```python
from build123d import *

# Parameters (mm, degrees)
F_35MM_DEPTH          = 35
CUT_EXTRUDE_1_REACH   = 50.244
SKETCH_2_R            = 10.5
FILLET_1_R            = 1
SKETCH_3_R            = 1.75
CUT_EXTRUDE_3_1_DEPTH = 35


with BuildPart() as part:
    # 草图1 → 高35mm (new body)
    with BuildSketch(Plane(origin=(0, 0, 0), x_dir=(1, 0, 0), z_dir=(0, 1, 0))):
        with BuildLine():
            Line((-20, 13.25250025), (-20, -7.909163894))
            ThreePointArc((-20, -7.909163894), (-19.67340752, -9.004475389), (-18.800292729, -9.742066387))
            ThreePointArc((-18.800292729, -9.742066387), (-16.040253129, -11.142625499), (-13.460543724, -12.852737719))
            ThreePointArc((-13.460543724, -12.852737719), (-12.893128183, -13.149929424), (-12.260860414, -13.25250025))
            Line((-12.260860414, -13.25250025), (12.260860414, -13.25250025))
            ThreePointArc((12.260860414, -13.25250025), (12.893128183, -13.149929424), (13.460543724, -12.852737719))
            ThreePointArc((13.460543724, -12.852737719), (16.040253129, -11.142625499), (18.800292729, -9.742066387))
            ThreePointArc((18.800292729, -9.742066387), (19.67340752, -9.004475389), (20, -7.909163894))
            Line((20, -7.909163894), (20, 13.25250025))
            Line((20, 13.25250025), (-20, 13.25250025))
        make_face()
    extrude(amount=F_35MM_DEPTH)

    # 草图2 → 切除-拉伸1 (cut, up to next)
    with BuildSketch(Plane(origin=(0, 0, -13.25250025), x_dir=(-1, 0, 0), z_dir=(0, 0, -1)), mode=Mode.PRIVATE) as cut_extrude_1_sk1:
        with Locations((0, 15)):
            Circle(SKETCH_2_R)
    cut_extrude_1_tool1 = extrude(cut_extrude_1_sk1.sketch, amount=-CUT_EXTRUDE_1_REACH, mode=Mode.PRIVATE) & part.part
    add(cut_extrude_1_tool1.solids().sort_by_distance((0, 15, -13.2525))[0], mode=Mode.SUBTRACT)

    # 圆角1
    fillet_1_edges = [part.edges().sort_by_distance(p)[0] for p in [
        (10.5, 15, -13.25250025),
        (10.5, 15, 13.25250025),
    ]]
    fillet(fillet_1_edges, radius=FILLET_1_R)

    # 草图3 → φ3.1通孔 (cut)
    with BuildSketch(Plane(origin=(0, 35, 0), x_dir=(1, 0, 0), z_dir=(0, 1, 0))):
        with Locations(Location((-15, 8.25250025, 0), (0, 0, 270))):
            Circle(SKETCH_3_R)
        with Locations(Location((-15, -6.74749975, 0), (0, 0, 270))):
            Circle(SKETCH_3_R)
        with Locations(Location((15, -6.74749975, 0), (0, 0, 90))):
            Circle(SKETCH_3_R)
        with Locations(Location((15, 8.25250025, 0), (0, 0, 90))):
            Circle(SKETCH_3_R)
    extrude(amount=-CUT_EXTRUDE_3_1_DEPTH, mode=Mode.SUBTRACT)


solid = part.part
```
Build history of the part. All positions in model axes, mm. Give positions to 0.01 mm unless a question says otherwise; leave off trailing zeros. Loops run counter-clockwise (first coordinate to the right, second up) from the corner with the lowest first, then second, coordinate; pieces in that order, holes last. Notation, with made-up numbers: (-37.5, 78.25) -> (10.5, 78.25) arc R20 ccw to (10.5, 82.25) -> close; hole circle Ø6 at (-3.5, 5). An arc over 180 degrees is marked (long way). One line per question, with ' | ' between items. Start each with the question number.
1) Cut at A-A (y = 15). Give the cut face in (x, z), plus the area to 3 significant figures.
2) Two-plate mould, pull along X, no slides. Class faces 1 (the cylindrical face through (-13.265, 17.745, 6.52)), 2 (the cylindrical face through (-19.682, 17.255, 8.991)), 3 (the flat face through (0, 29, -13.253)), 4 (the flat face through (20, 17, -3)): released by +X, released by -X, zero draft, split by the parting line, or undercut.
3) Cut at C-C (z = -1). Give the cut face in (x, y), plus the area to 3 significant figures.
4) Cut at B-B (x = 0). Give the cut face in (y, z).
5) Cut at D-D (x = 15). Give the cut face in (y, z), plus the area to 3 significant figures.
6) Pin check, flat tip, straight feed: pin 1 (17 mm diameter, centred on x = 0, y = 15, fed in from +Z). Stop position of the tip, or through.
7) Probe L1, parallel to X at y = 8.5, z = -9; L2, parallel to Z at x = 15, y = 22; L3, parallel to Z at x = 14.5, y = 24. List the from-to ranges inside material, lowest first.
Return value:
1) outline: (-20, -13.25) -> (-11.5, -13.25) arc R1 ccw to (-10.5, -12.25) -> (-10.5, 12.25) arc R1 ccw to (-11.5, 13.25) -> (-12.26, 13.25) arc R2 ccw to (-13.46, 12.85) arc R26.74 cw to (-18.8, 9.74) arc R2 ccw to (-20, 7.91) -> close; (10.5, -12.25) arc R1 ccw to (11.5, -13.25) -> (20, -13.25) -> (20, 7.91) arc R2 ccw to (18.8, 9.74) arc R26.74 cw to (13.46, 12.85) arc R2 ccw to (12.26, 13.25) -> (11.5, 13.25) arc R1 ccw to (10.5, 12.25) -> close; hole circle Ø3.5 at (-15, -8.25); hole circle Ø3.5 at (-15, 6.75); hole circle Ø3.5 at (15, -8.25); hole circle Ø3.5 at (15, 6.75) | area: 432 mm^2
2) face 1: undercut | face 2: released by -X | face 3: zero draft | face 4: released by +X
3) outline: (-20, 0) -> (20, 0) -> (20, 35) -> (-20, 35) -> close; hole circle Ø21 at (0, 15) | area: 1,050 mm^2
4) outline: (0, -13.25) -> (3.5, -13.25) arc R1 ccw to (4.5, -12.25) -> (4.5, 12.25) arc R1 ccw to (3.5, 13.25) -> (0, 13.25) -> close; (25.5, -12.25) arc R1 ccw to (26.5, -13.25) -> (35, -13.25) -> (35, 13.25) -> (26.5, 13.25) arc R1 ccw to (25.5, 12.25) -> close
5) outline: (0, -13.25) -> (35, -13.25) -> (35, -10) -> (0, -10) -> close; (0, -6.5) -> (35, -6.5) -> (35, 5) -> (0, 5) -> close; (0, 8.5) -> (35, 8.5) -> (35, 11.78) -> (0, 11.78) -> close | area: 631 mm^2
6) pin 1: through
7) L1: -20 to -16.58, -13.42 to -8.25, 8.25 to 13.42, 16.58 to 20 | L2: -13.25 to -10, -6.5 to 5, 8.5 to 11.78 | L3: -13.25 to -9.93, -6.58 to 5.07, 8.42 to 12.11
